Autodesk Inventor part; units mm, degrees
ref_plane "YZ Plane" through (0, 0, 0) normal (1, 0, 0) x (0, 1, 0)
ref_plane "XZ Plane" through (0, 0, 0) normal (0, 1, 0) x (-1, 0, 0)
ref_plane "XY Plane" through (0, 0, 0) normal (0, 0, 1) x (1, 0, 0)
sketch "草圖1" plane through (0, 0, 0) normal (0, 0, 1) x (1, 0, 0)
  line L0 (0, 0) -> (0, 12.55)
  line L1 (0, 12.55) -> (-29.22, 12.55)
  line L2 (-29.22, 12.55) -> (-29.22, 4.75)
  line L3 (-29.22, 4.75) -> (-144.22, 4.75)
  line L4 (-144.22, 4.75) -> (-144.22, 0)
  line L5 (-144.22, 0) -> (0, 0)
  dimension "d0" = 29.22
  dimension "d1" = 12.55
  dimension "d2" = 115
  dimension "d3" = 4.75
revolve "迴轉1" add sketch "草圖1" angle 360 about axis through (-144.22, 0, 0) along (1, 0, 0)
chamfer "倒角1" distance 1 angle 45 1 edges at (-144.22, -4.75, 0)
thread "螺紋1"
sketch "草圖2" plane through (-144.22, 0, 0) normal (-1, 0, 0) x (0, 0, 1)
  circle A0 centre (0, 0) radius 2
  dimension "d10" = 4
extrude "擠出1" cut sketch "草圖2" against normal blind 3.8
properties part number "螺桿" material "鋁合金 6061"
Read the model definition and answer for the solid it produces. Units are mm, in the model's axes. A direction names the side the tool comes from. Give positions to 0.01 mm unless a question says otherwise; leave off trailing zeros. Write each loop counter-clockwise with the first axis right and the second up, starting at its lowest first coordinate (ties: lowest second). Pieces come first, ordered by that corner, then holes. Notation, with made-up numbers: M 4.25,-30 L 47.25,-30 A15 ccw 47.25,-17 Z; hole C -39.5,50 d11. An arc over 180 degrees is marked long. One line per item, written item: value. Start each with the question number.
(1) Find the intervals of material crossed by line 1 (X direction, y = 1.75, z = -10.5); line 2 (Y direction, x = -143.35, z = 0); line 3 (Y direction, x = -84.5, z = 2.5), in increasing order.
(2) Find section C-C (x = -109). Determine the outline of the cut face in (y, z).
(3) A tool of negligible diameter and unlimited length cuts with its end or side. For faces 5 (the cylindrical face through (-87.018, 2.192, 4.214)), 6 (the flat face through (-144.22, 2, -2)), from which of +Z, -Z, +X, -X, +Y, -Y can it reach the whole face along a straight path? Write none if from no direction.
(4) Determine the mould class of faces 1 (the flat face through (0, 0, 0)), 2 (the flat face through (-140.42, 0, 0)), 3 (the cylindrical face through (-14.81, 11.59, 4.81)), 4 (the cylindrical face through (-142, -2, 0)) for opening direction Z: pulls with the +Z half, pulls with the -Z half, needs draft (parallel to the pull), parting line crosses it, or undercut.
(5) Find section D-D (x = -21). Determine the outline of the cut face in (y, z), plus the area to 3 significant figures.
(6) Flat-ended cylindrical pins translate along their axes: pin 1 Ø10 at (x, y) = (-63.5, -5.5) entering from -Z; pin 2 Ø3.5 at (y, z) = (0, 0) entering from -X; pin 3 Ø1 at (x, y) = (-125, 3.5) entering from -Z. Find the tip coordinate at first contact, or state that the pin passes through.
(7) Find section A-A (y = 0). Determine the outline of the cut face in (x, z), plus the area to 3 significant figures.
Results below:
1. line 1: x = -29.22 to 0
1. line 2: y = -4.62 to -2, 2 to 4.62
1. line 3: y = -4.04 to 4.04
2. outline: C 0,0 d9.5
3. face 5: -X
3. face 6: +Z, -Z, -X, +Y, -Y
4. face 1: needs draft
4. face 2: undercut
4. face 3: parting line crosses it
4. face 4: undercut
5. outline: C 0,0 d25.1
5. area: 495 mm^2
6. pin 1: stops at z = -4.72
6. pin 2: stops at x = -140.42
6. pin 3: stops at z = -3.68
7. outline: M -144.22,-3.75 L -143.22,-4.75 L -29.22,-4.75 L -29.22,-12.55 L 0,-12.55 L 0,12.55 L -29.22,12.55 L -29.22,4.75 L -143.22,4.75 L -144.22,3.75 L -144.22,2 L -140.42,2 L -140.42,-2 L -144.22,-2 Z
7. area: 1,810 mm^2
